from build123d import *

# Parameters (mm, degrees)
F1_DEPTH = 8
F2_W     = 3.703703
F2_H     = 20
F3_DEPTH = 9.30533


with BuildPart() as f1:
    # F0 (on Right) → F1 (new body)
    with BuildSketch(Plane.YZ):
        with BuildLine():
            Line((18.307374, 8.89), (-6.457626, 8.89))
            ThreePointArc((-6.457626, 8.89), (-6.906639, 8.704013), (-7.092626, 8.255))
            Line((-7.092626, 8.255), (-7.092626, 0))
            Line((-7.092626, 0), (18.307374, 0))
            Line((18.307374, 0), (18.307374, 8.89))
        make_face()
    extrude(amount=F1_DEPTH)

    # F2 (on Top) → F3 (cut)
    with BuildSketch(Plane.XY):
        with Locations((4.075629, -0.084073)):
            Rectangle(F2_W, F2_H)
    extrude(amount=F3_DEPTH, mode=Mode.SUBTRACT)


solid = f1.part
Work out the finished part from the listing and answer in its coordinate system (mm). A direction names the side the tool comes from. Give positions to 0.01 mm unless a question says otherwise; leave off trailing zeros. Write each loop counter-clockwise with the first axis right and the second up, starting at its lowest first coordinate (ties: lowest second). Pieces come first, ordered by that corner, then holes. Notation, with made-up numbers: (20.25, 44) - (31.25, 44) arc R26 ccw to (31.25, 76) - close; hole circle Ø7 at (-34.5, 21). An arc over 180 degrees is marked (long way). One line per item, written item: value. Start each with the question number.
1. For faces 4 (the flat face through (2, 9, 8.89)), 5 (the flat face through (4, 9.916, 4)), determine the directions among +Z, -Z, +X, -X, +Y, -Y from which every point of the face is accessible in a straight line to the end or side of a thin tool.
2. Find section C-C (x = 2.5). Write down the section's boundary in (y, z).
3. Given pin 1 (1 mm diameter, centred on x = 4, z = 7, fed in from -Y), flat-ended and moving along its own axis, determine where the tip first touches the part or whether it passes through.
4. Find section A-A (y = 2.75). Write down the section's boundary in (x, z), then the cut area to 3 significant figures.
5. Consider probe 1 along X at (y, z) = (1.25, 1); probe 2 along Y at (x, z) = (2.75, 3.5). Determine where each line is inside the solid, lowest interval first.
6. For a pull along X with two mould halves and no side action, classify faces 1 (the flat face through (8, 5, 5)), 2 (the flat face through (4, 18.307, 4)), 3 (the flat face through (2.224, 1, 4)) as +X half, -X half, draft (parallel to the pull), parting line (faces both ways), or undercut.
7. Find section B-B (z = 2.5). Write down the section's boundary in (x, y), then the cut area to 3 significant figures.
Geometry results:
1. face 4: +Z, +X, -X, +Y, -Y
1. face 5: +Z, -Z, -Y
2. outline: (9.92, 0) - (18.31, 0) - (18.31, 8.89) - (9.92, 8.89) - close
3. pin 1: y = 9.92
4. outline: (0, 0) - (2.22, 0) - (2.22, 8.89) - (0, 8.89) - close; (5.93, 0) - (8, 0) - (8, 8.89) - (5.93, 8.89) - close
4. area: 38.2 mm2
5. probe 1: 0 to 2.22, 5.93 to 8
5. probe 2: 9.92 to 18.31
6. face 1: +X half
6. face 2: draft
6. face 3: undercut
7. outline: (0, -7.09) - (2.22, -7.09) - (2.22, 9.92) - (5.93, 9.92) - (5.93, -7.09) - (8, -7.09) - (8, 18.31) - (0, 18.31) - close
7. area: 140 mm2
